Can you work these out from the model? Positions are in its coordinate system, mm. Face numbers are marked on the shaded views. A direction names the side the tool comes from. Round coordinates to 2 decimals unless told otherwise and drop trailing zeros. Order: outer loops, then holes, each group sorted by start corner. A loop starts at its lowest first (then second) coordinate and runs counter-clockwise, first axis right, second up.
Q1. Will these pins go through, and if not, where does the flat tip stop? P1, Ø12, axis at x = -44.5, z = 9, coming from the -Y side; P2, Ø1.6, axis at y = 1.5, z = -29.5, coming from the +X side; P3, Ø4, axis at x = 35, z = -27.5, coming from the +Y side; P4, Ø4, axis at y = 42, z = 26.5, coming from the -X side.
Q2. If we section it at B-B (z = 27.5): Please give me the cut outline in (x, y).
Q3. We'd pull the mould along Z, two halves only. Please class the marked faces 3, 4 and 5: pulls with the +Z half, pulls with the -Z half, needs draft (parallel to the pull), parting line crosses it, or undercut.
Q4. If we section it at C-C (y = 9): Please give me the cut outline in (x, z), plus the area to 3 significant figures.
Q5. If I drill on line 1 (Z direction, x = 35, y = 0.7); line 2 (X direction, y = 0.6, z = 27.5); line 3 (X direction, y = 38.5, z = 25), over which ranges is the centre line in solid material (lowest first)?
Q6. For the marked faces 1 and 2, which set-ups out of +Z, -Z, +X, -X, +Y, -Y let a thin tool reach every point of the face, with its end or its side?
Q7. If we section it at A-A (x = -20): Please give me the cut outline in (y, z).
Q8. If we section it at D-D (x = 35): Please give me the cut outline in (y, z), plus the area to 3 significant figures.
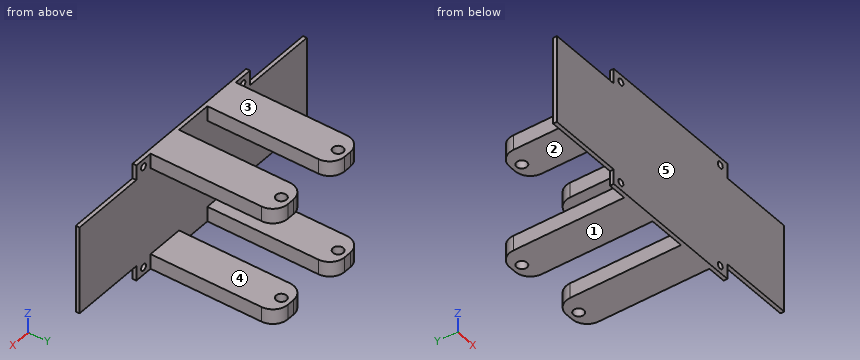
from build123d import *

# Parameters (mm, degrees)
SKETCH_1_R               = 1.75
EXTRUDE_1_DEPTH          = 2
SKETCH_2_W               = 20
SKETCH_2_H               = 8
EXTRUDE_2_DEPTH          = 67
SKETCH_3_R               = 2.75
CUT_EXTRUDE_1_DEPTH      = 1
CUT_EXTRUDE_1_DEPTH_BACK = 64
FILLET_1_R               = 8


with BuildPart() as part:
    # Эскиз1 → Бобышка-Вытянуть1 (new body)
    with BuildSketch(Plane(origin=(0, 0, 0), x_dir=(1, 0, 0), z_dir=(0, 1, 0))):
        Polygon((-80, -23.5), (-40, -23.5), (-40, -31.5), (40, -31.5), (40, -23.5), (80, -23.5), (80, 23.5), (40, 23.5), (40, 31.5), (-40, 31.5), (-40, 23.5), (-80, 23.5), align=None)
        with Locations((-35, 27.5)):
            Circle(SKETCH_1_R, mode=Mode.SUBTRACT)
        with Locations((35, 27.5)):
            Circle(SKETCH_1_R, mode=Mode.SUBTRACT)
        with Locations((35, -27.5)):
            Circle(SKETCH_1_R, mode=Mode.SUBTRACT)
        with Locations((-35, -27.5)):
            Circle(SKETCH_1_R, mode=Mode.SUBTRACT)
    extrude(amount=EXTRUDE_1_DEPTH)

    # Эскиз2 → Бобышка-Вытянуть2 (add)
    with BuildSketch(Plane(origin=(0, 2, 0), x_dir=(1, 0, 0), z_dir=(0, 1, 0))):
        with Locations((20, -27.5)):
            Rectangle(SKETCH_2_W, SKETCH_2_H)
        with Locations((-20, -27.5)):
            Rectangle(SKETCH_2_W, SKETCH_2_H)
        with Locations((20, 27.5)):
            Rectangle(SKETCH_2_W, SKETCH_2_H)
        with Locations((-20, 27.5)):
            Rectangle(SKETCH_2_W, SKETCH_2_H)
    extrude(amount=EXTRUDE_2_DEPTH)

    # Эскиз3 → Вырез-Вытянуть1 (cut, two sides)
    with BuildSketch(Plane.XY.offset(31.5)) as cut_extrude_1_sk:
        with Locations((-20, 64)):
            Circle(SKETCH_3_R)
        with Locations((20, 64)):
            Circle(SKETCH_3_R)
    extrude(amount=CUT_EXTRUDE_1_DEPTH, mode=Mode.SUBTRACT)
    extrude(cut_extrude_1_sk.sketch, amount=-CUT_EXTRUDE_1_DEPTH_BACK, mode=Mode.SUBTRACT)

    # Скругление1
    fillet_1_edges = [part.edges().sort_by_distance(p)[0] for p in [
        (-30, 69, 27.5),
        (-10, 69, 27.5),
        (30, 69, 27.5),
        (10, 69, 27.5),
        (10, 69, -27.5),
        (30, 69, -27.5),
        (-30, 69, -27.5),
        (-10, 69, -27.5),
    ]]
    fillet(fillet_1_edges, radius=FILLET_1_R)


solid = part.part
Solution:
1. P1: stops at y = 0
1. P2: stops at x = 40
1. P3: stops at y = 2
1. P4: stops at x = -30
2. outline: (-40, 0) - (-36.75, 0) - (-36.75, 2) - (-40, 2) - close; (-33.25, 0) - (33.25, 0) - (33.25, 2) - (30, 2) - (30, 61) arc R8 ccw to (22, 69) - (18, 69) arc R8 ccw to (10, 61) - (10, 2) - (-10, 2) - (-10, 61) arc R8 ccw to (-18, 69) - (-22, 69) arc R8 ccw to (-30, 61) - (-30, 2) - (-33.25, 2) - close; (36.75, 0) - (40, 0) - (40, 2) - (36.75, 2) - close; hole circle Ø5.5 at (-20, 64); hole circle Ø5.5 at (20, 64)
3. face 3: pulls with the +Z half
3. face 4: undercut
3. face 5: needs draft
4. outline: (-30, -31.5) - (-10, -31.5) - (-10, -23.5) - (-30, -23.5) - close; (-30, 23.5) - (-10, 23.5) - (-10, 31.5) - (-30, 31.5) - close; (10, -31.5) - (30, -31.5) - (30, -23.5) - (10, -23.5) - close; (10, 23.5) - (30, 23.5) - (30, 31.5) - (10, 31.5) - close
4. area: 640 mm2
5. line 1: z = -31.5 to -29.25, -25.75 to 25.75, 29.25 to 31.5
5. line 2: x = -40 to -36.75, -33.25 to 33.25, 36.75 to 40
5. line 3: x = -30 to -10, 10 to 30
6. face 1: -Z, +X, -X, +Y, -Y
6. face 2: +X, -X, +Y
7. outline: (0, -31.5) - (61.25, -31.5) - (61.25, -23.5) - (2, -23.5) - (2, 23.5) - (61.25, 23.5) - (61.25, 31.5) - (0, 31.5) - close; (66.75, -31.5) - (69, -31.5) - (69, -23.5) - (66.75, -23.5) - close; (66.75, 23.5) - (69, 23.5) - (69, 31.5) - (66.75, 31.5) - close
8. outline: (0, -31.5) - (2, -31.5) - (2, -29.25) - (0, -29.25) - close; (0, -25.75) - (2, -25.75) - (2, 25.75) - (0, 25.75) - close; (0, 29.25) - (2, 29.25) - (2, 31.5) - (0, 31.5) - close
8. area: 112 mm2
